Read the model definition and answer for the solid it produces. Units are mm, in the model's axes. A direction names the side the tool comes from. Give positions to 0.01 mm unless a question says otherwise; leave off trailing zeros. Write each loop counter-clockwise with the first axis right and the second up, starting at its lowest first coordinate (ties: lowest second). Pieces come first, ordered by that corner, then holes. Notation, with made-up numbers: (-5, 57.5) -> (53, 57.5) arc R11 ccw to (53, 70.5) -> close; hole circle Ø8 at (30, 55). An arc over 180 degrees is marked (long way). Use a Markdown table: item, result.
from build123d import *

# Parameters (mm, degrees)
BOSS_EXTRUDE1_DEPTH = 10
FILLET1_R           = 10
SKETCH2_W           = 40
SKETCH2_H           = 2
BOSS_EXTRUDE2_DEPTH = 75
FILLET2_R           = 5
CUT_EXTRUDE1_REACH  = 219.69
SKETCH4_R           = 5.5


with BuildPart() as part:
    # Sketch1 → Boss-Extrude1 (new, symmetric)
    with BuildSketch(Plane.XY):
        Polygon((0, 0), (-50, 0), (-50, -40), (-100, -40), (-100, -38), (-52, -38), (-52, 2), (0, 2), align=None)
    extrude(amount=BOSS_EXTRUDE1_DEPTH, both=True)

    # Fillet1
    fillet1_edges = [part.edges().sort_by_distance(p)[0] for p in [
        (-50, 0, 0),
        (-50, -40, 0),
        (-52, -38, 0),
        (-52, 2, 0),
    ]]
    fillet(fillet1_edges, radius=FILLET1_R)

    # Sketch2 → Boss-Extrude2 (add, symmetric)
    with BuildSketch(Plane.XY):
        with Locations((-20, 1)):
            Rectangle(SKETCH2_W, SKETCH2_H)
    extrude(amount=BOSS_EXTRUDE2_DEPTH, both=True)

    # Fillet2
    fillet2_edges = [part.edges().sort_by_distance(p)[0] for p in [
        (-40, 1, -75),
        (0, 1, -75),
        (-40, 1, 75),
        (0, 1, 75),
    ]]
    fillet(fillet2_edges, radius=FILLET2_R)

    # Mirror1: part across plane


with BuildPart() as part_1:
    add(part.part)
    add(part.part.mirror(Plane(origin=(-100, -38, 10), x_dir=(0, 0, 1), z_dir=(1, 0, 0))))

    # Sketch4 → Cut-Extrude1 (cut, up to next)
    with BuildSketch(Plane.XZ.offset(40), mode=Mode.PRIVATE) as cut_extrude1_sk1:
        with Locations((-100, 0)):
            Circle(SKETCH4_R)
    cut_extrude1_tool1 = extrude(cut_extrude1_sk1.sketch, amount=-CUT_EXTRUDE1_REACH, mode=Mode.PRIVATE) & part_1.part
    add(cut_extrude1_tool1.solids().sort_by_distance((-100, -40, 0))[0], mode=Mode.SUBTRACT)


solid = part_1.part
Item 1: Each of these flat-tipped pins is pushed along its axis until it touches: P1, Ø22, axis at y = -22, z = 0.5, coming from the -X side; P2, Ø10, axis at y = -17.5, z = 3.5, coming from the +X side; P3, Ø22, axis at y = -19.5, z = -4.5, coming from the -X side; P4, Ø10, axis at x = -113, y = -29.5, coming from the -Z side. Where does it stop, or does it pass through?
Return value:
| item | result |
|---|---|
| P1 | x = -150 |
| P2 | x = -50 |
| P3 | x = -150.11 |
| P4 | through |
Item 2: A cutting plane is placed at D-D (x = -66.5). Give the vertices of the cut face in (y, z), then the cut area to 3 significant figures.
Return value:
| item | result |
|---|---|
| outline | (-40, -10) -> (-38, -10) -> (-38, 10) -> (-40, 10) -> close |
| area | 40.0 mm^2 |
Item 3: A cutting plane is placed at C-C (y = -14.5). Give the vertices of the cut face in (x, z), then the cut area to 3 significant figures.
Return value:
| item | result |
|---|---|
| outline | (-150, -10) -> (-148, -10) -> (-148, 10) -> (-150, 10) -> close; (-52, -10) -> (-50, -10) -> (-50, 10) -> (-52, 10) -> close |
| area | 80.0 mm^2 |
Item 4: For a pull along X with two mould halves and no side action, classify faces 4 (the face through (-48.99, -0.85, 0.14)), 5 (the face through (-199, 1, 73)), 6 (the face through (-179, 2, 1)) as +X half, -X half, draft (parallel to the pull), parting line (faces both ways), or undercut.
Return value:
| item | result |
|---|---|
| face 4 | undercut |
| face 5 | -X half |
| face 6 | draft |
Item 5: Straight lines are drawn through the part: line 1 along Z through (x, y) = (-100, -39.3); line 2 along X through (y, z) = (0.5, 44); line 3 along X through (y, z) = (-27.5, 3.5). For each, find the intervals that lie inside material, in ascending order. Write a range as [from, to].
Return value:
| item | result |
|---|---|
| line 1 | [-10, -5.5], [5.5, 10] |
| line 2 | [-200, -160], [-40, 0] |
| line 3 | [-150, -148], [-52, -50] |
Item 6: A cutting plane is placed at A-A (x = -100). Give the vertices of the cut face in (y, z), then the cut area to 3 significant figures.
Return value:
| item | result |
|---|---|
| outline | (-40, -10) -> (-38, -10) -> (-38, -5.5) -> (-40, -5.5) -> close; (-40, 5.5) -> (-38, 5.5) -> (-38, 10) -> (-40, 10) -> close |
| area | 18.0 mm^2 |
Item 7: A cutting plane is placed at B-B (z = 0). Give the vertices of the cut face in (x, y), then the cut area to 3 significant figures.
Return value:
| item | result |
|---|---|
| outline | (-200, 0) -> (-160, 0) arc R10 cw to (-150, -10) -> (-150, -30) arc R10 ccw to (-140, -40) -> (-105.5, -40) -> (-105.5, -38) -> (-138, -38) arc R10 cw to (-148, -28) -> (-148, -8) arc R10 ccw to (-158, 2) -> (-200, 2) -> close; (-94.5, -40) -> (-60, -40) arc R10 ccw to (-50, -30) -> (-50, -10) arc R10 cw to (-40, 0) -> (0, 0) -> (0, 2) -> (-42, 2) arc R10 ccw to (-52, -8) -> (-52, -28) arc R10 cw to (-62, -38) -> (-94.5, -38) -> close |
| area | 538 mm^2 |
Item 8: A tool of negligible diameter and unlimited length cuts with its end or side. For faces 1 (the face through (-38, 1, 74)), 2 (the face through (-151.01, -0.85, 0.14)), 3 (the face through (-161, 1, -73)), from which of +Z, -Z, +X, -X, +Y, -Y can it reach the whole face along a straight path? Write none if from no direction.
Return value:
| item | result |
|---|---|
| face 1 | +Z, +Y, -Y |
| face 2 | +Z, -Z, +Y |
| face 3 | -Z, +Y, -Y |
